from build123d import *

# Parameters (mm, degrees)
F1_DEPTH = 152.4


with BuildPart() as f1:
    # F0 (on Front) → F1 (new body)
    with BuildSketch(Plane.XZ):
        with BuildLine():
            Line((-1.056078, 0.150868), (0, 0))
            Line((0, 0), (36.542293, 255.796051))
            ThreePointArc((36.542293, 255.796051), (40.793589, 263.594265), (49.114652, 266.7))
            Line((49.114652, 266.7), (68.207103, 266.7))
            ThreePointArc((68.207103, 266.7), (76.156388, 266.284226), (84.018924, 265.04144))
            Line((84.018924, 265.04144), (487.121544, 179.534824))
            ThreePointArc((487.121544, 179.534824), (493.518553, 176.039147), (496.939615, 169.601926))
            Line((496.939615, 169.601926), (497.199711, 168.301447))
            ThreePointArc((497.199711, 168.301447), (506.851257, 152.974208), (524.260375, 147.974287))
            Line((524.260375, 147.974287), (788.147179, 170.432739))
            ThreePointArc((788.147179, 170.432739), (797.130539, 167.717236), (801.796495, 159.574535))
            Line((801.796495, 159.574535), (825.5, -6.35))
            Line((825.5, -6.35), (826.556078, -6.199132))
            Line((826.556078, -6.199132), (802.852573, 159.725403))
            ThreePointArc((802.852573, 159.725403), (797.794677, 168.552091), (788.056714, 171.495696))
            Line((788.056714, 171.495696), (524.169911, 149.037245))
            ThreePointArc((524.169911, 149.037245), (507.491976, 153.827168), (498.245794, 168.510664))
            Line((498.245794, 168.510664), (497.985698, 169.811142))
            ThreePointArc((497.985698, 169.811142), (494.277267, 176.78909), (487.342909, 180.578404))
            Line((487.342909, 180.578404), (84.24029, 266.08502))
            ThreePointArc((84.24029, 266.08502), (76.267678, 267.345205), (68.207103, 267.7668))
            Line((68.207103, 267.7668), (49.114652, 267.7668))
            ThreePointArc((49.114652, 267.7668), (40.09462, 264.400184), (35.486215, 255.94692))
            Line((35.486215, 255.94692), (-1.056078, 0.150868))
        make_face()
    extrude(amount=F1_DEPTH)


solid = f1.part
Geometry: final body of the model. Coordinates: model frame, mm. A direction names the side the tool comes from. Give positions to 0.01 mm unless a question says otherwise; leave off trailing zeros. Write each loop counter-clockwise with the first axis right and the second up, starting at its lowest first coordinate (ties: lowest second). Pieces come first, ordered by that corner, then holes.
(1) Cut plane D-D, the plane x = 134. Return loops of the section in (y, z), then the cut area to 3 significant figures.
(2) Access query for faces 1 (the flat face through (17.47, -75.13, 129.84)), 2 (the flat face through (18, -75, 126)), 3 (the flat face through (657.961, -75.133, 160.424)). Directions: +Z, -Z, +X, -X, +Y, -Y. A direction counts if a zero-diameter tool reaches every point of the face in a straight line with its end or side. Return the directions, or none.
(3) Cut plane B-B, the plane y = -83.5. Return loops of the section in (x, z).
(4) First-contact query: P1, Ø1.5, axis at y = -29.5, z = 45.5, coming from the -X side; P2, Ø9.5, axis at x = 60.5, y = -82.5, coming from the -Z side; P3, Ø2, axis at y = -64, z = 76.5, coming from the +X side. Flat tips, straight axial feed; report the tip coordinate or a pass-through.
(5) Cut plane C-C, the plane z = 96. Return loops of the section in (x, y).
(6) Cut plane A-A, the plane z = 237.5. Return loops of the section in (x, y).
(7) Ray query, line 1 (X direction, y = -77.5, z = 90); line 2 (X direction, y = -121, z = 38); line 3 (Z direction, x = 723, y = -110.5). Return the intervals inside material, ascending.
(8) Mould query, pull axis X, two halves, no side actions, for faces 4 (the cylindrical face through (76, -75.1, 266.3)), 5 (the cylindrical face through (40.2, -75.13, 264.49)), 6 (the flat face through (814.87, -75.13, 75.6)). Classes: released by +X, released by -X, zero draft, split by the parting line, or undercut.
Values follow:
1. outline: (-152.4, 254.44) - (0, 254.44) - (0, 255.53) - (-152.4, 255.53) - close
1. area: 166 mm2
2. face 1: +Z, -X, +Y, -Y
2. face 2: -Z, +Y, -Y
2. face 3: +Z, +Y, -Y
3. outline: (-1.06, 0.15) - (0, 0) - (36.54, 255.8) arc R12.7 cw to (49.11, 266.7) - (68.21, 266.7) arc R76.2 cw to (84.02, 265.04) - (487.12, 179.53) arc R12.7 cw to (496.94, 169.6) - (497.2, 168.3) arc R25.4 ccw to (524.26, 147.97) - (788.15, 170.43) arc R12.7 cw to (801.8, 159.57) - (825.5, -6.35) - (826.56, -6.2) - (802.85, 159.73) arc R13.77 ccw to (788.06, 171.5) - (524.17, 149.04) arc R24.33 cw to (498.25, 168.51) - (497.99, 169.81) arc R13.77 ccw to (487.34, 180.58) - (84.24, 266.09) arc R77.27 ccw to (68.21, 267.77) - (49.11, 267.77) arc R13.77 ccw to (35.49, 255.95) - close
4. P1: stops at x = 5.32
4. P2: stops at z = 266.7
4. P3: stops at x = 814.88
5. outline: (12.64, -152.4) - (13.71, -152.4) - (13.71, 0) - (12.64, 0) - close; (810.88, -152.4) - (811.96, -152.4) - (811.96, 0) - (810.88, 0) - close
6. outline: (32.85, -152.4) - (33.93, -152.4) - (33.93, 0) - (32.85, 0) - close; (213.86, -152.4) - (219, -152.4) - (219, 0) - (213.86, 0) - close
7. line 1: x = 11.78 to 12.86, 811.74 to 812.81
7. line 2: x = 4.35 to 5.43, 819.16 to 820.24
7. line 3: z = 164.89 to 165.96
8. face 4: undercut
8. face 5: released by -X
8. face 6: released by +X
